from build123d import *

# Parameters (mm, degrees)
MODEL_W            = 2.54
MODEL_H            = 30.48
MODEL_H_2          = 20.32
MODEL_W_2          = 5.08
MODEL_H_3          = 5.08
BOSS_EXTRU_1_DEPTH = 1.5


with BuildPart() as part:
    # Model → Boss.-Extru.1 (new body)
    with BuildSketch(Plane.XY):
        with BuildLine():
            Line((110.49, -34.813931), (110.49, -38.623931))
            Line((110.49, -38.623931), (110.49, -39.893931))
            Line((110.49, -39.893931), (110.49, -123.713931))
            add(Edge.make_bspline(
                [(109.746051, -125.509982), (110.222394, -125.03364), (110.49, -124.387581), (110.49, -123.713931)],
                knots=[0, 0, 0, 0, 1, 1, 1, 1], degree=3))
            add(Edge.make_bspline(
                [(107.95, -126.253931), (108.62365, -126.253931), (109.269709, -125.986325), (109.746051, -125.509982)],
                knots=[0, 0, 0, 0, 1, 1, 1, 1], degree=3))
            Line((107.95, -126.253931), (85.09, -126.253931))
            add(Edge.make_bspline(
                [(83.293949, -125.509982), (83.770291, -125.986325), (84.41635, -126.253931), (85.09, -126.253931)],
                knots=[0, 0, 0, 0, 1, 1, 1, 1], degree=3))
            add(Edge.make_bspline(
                [(82.55, -123.713931), (82.55, -124.387581), (82.817606, -125.03364), (83.293949, -125.509982)],
                knots=[0, 0, 0, 0, 1, 1, 1, 1], degree=3))
            Line((82.55, -123.713931), (82.55, -39.893931))
            Line((82.55, -39.893931), (82.55, -38.623931))
            Line((82.55, -38.623931), (82.55, -34.813931))
            add(Edge.make_bspline(
                [(82.921974, -33.915905), (82.683803, -34.154076), (82.55, -34.477106), (82.55, -34.813931)],
                knots=[0, 0, 0, 0, 1, 1, 1, 1], degree=3))
            add(Edge.make_bspline(
                [(83.82, -33.543931), (83.483175, -33.543931), (83.160146, -33.677734), (82.921974, -33.915905)],
                knots=[0, 0, 0, 0, 1, 1, 1, 1], degree=3))
            Line((83.82, -33.543931), (109.22, -33.543931))
            add(Edge.make_bspline(
                [(110.118026, -33.915905), (109.879854, -33.677734), (109.556825, -33.543931), (109.22, -33.543931)],
                knots=[0, 0, 0, 0, 1, 1, 1, 1], degree=3))
            add(Edge.make_bspline(
                [(110.49, -34.813931), (110.49, -34.477106), (110.356197, -34.154076), (110.118026, -33.915905)],
                knots=[0, 0, 0, 0, 1, 1, 1, 1], degree=3))
        make_face()
        with Locations((107.95, -95.138931)):
            Rectangle(MODEL_W, MODEL_H, mode=Mode.SUBTRACT)
        with Locations((85.09, -90.058931)):
            Rectangle(MODEL_W, MODEL_H_2, mode=Mode.SUBTRACT)
        with Locations((93.98, -105.933931)):
            Rectangle(MODEL_W_2, MODEL_H_3, mode=Mode.SUBTRACT)
        with BuildLine():
            add(Edge.make_bspline(
                [(109.22, -36.083931), (109.22, -36.537658), (108.977939, -36.956919), (108.585, -37.183783)],
                knots=[0, 0, 0, 0, 1, 1, 1, 1], degree=3))
            add(Edge.make_bspline(
                [(108.585, -37.183783), (108.192061, -37.410647), (107.707939, -37.410647), (107.315, -37.183783)],
                knots=[0, 0, 0, 0, 1, 1, 1, 1], degree=3))
            add(Edge.make_bspline(
                [(107.315, -37.183783), (106.922061, -36.956919), (106.68, -36.537658), (106.68, -36.083931)],
                knots=[0, 0, 0, 0, 1, 1, 1, 1], degree=3))
            add(Edge.make_bspline(
                [(106.68, -36.083931), (106.68, -35.630204), (106.922061, -35.210942), (107.315, -34.984079)],
                knots=[0, 0, 0, 0, 1, 1, 1, 1], degree=3))
            add(Edge.make_bspline(
                [(107.315, -34.984079), (107.707939, -34.757215), (108.192061, -34.757215), (108.585, -34.984079)],
                knots=[0, 0, 0, 0, 1, 1, 1, 1], degree=3))
            add(Edge.make_bspline(
                [(108.585, -34.984079), (108.977939, -35.210942), (109.22, -35.630204), (109.22, -36.083931)],
                knots=[0, 0, 0, 0, 1, 1, 1, 1], degree=3))
        make_face(mode=Mode.SUBTRACT)
        with BuildLine():
            add(Edge.make_bspline(
                [(86.36, -36.083931), (86.36, -36.537658), (86.117939, -36.956919), (85.725, -37.183783)],
                knots=[0, 0, 0, 0, 1, 1, 1, 1], degree=3))
            add(Edge.make_bspline(
                [(85.725, -37.183783), (85.332061, -37.410647), (84.847939, -37.410647), (84.455, -37.183783)],
                knots=[0, 0, 0, 0, 1, 1, 1, 1], degree=3))
            add(Edge.make_bspline(
                [(84.455, -37.183783), (84.062061, -36.956919), (83.82, -36.537658), (83.82, -36.083931)],
                knots=[0, 0, 0, 0, 1, 1, 1, 1], degree=3))
            add(Edge.make_bspline(
                [(83.82, -36.083931), (83.82, -35.630204), (84.062061, -35.210942), (84.455, -34.984079)],
                knots=[0, 0, 0, 0, 1, 1, 1, 1], degree=3))
            add(Edge.make_bspline(
                [(84.455, -34.984079), (84.847939, -34.757215), (85.332061, -34.757215), (85.725, -34.984079)],
                knots=[0, 0, 0, 0, 1, 1, 1, 1], degree=3))
            add(Edge.make_bspline(
                [(85.725, -34.984079), (86.117939, -35.210942), (86.36, -35.630204), (86.36, -36.083931)],
                knots=[0, 0, 0, 0, 1, 1, 1, 1], degree=3))
        make_face(mode=Mode.SUBTRACT)
        with BuildLine():
            add(Edge.make_bspline(
                [(86.36, -123.713931), (86.36, -124.167658), (86.117939, -124.586919), (85.725, -124.813783)],
                knots=[0, 0, 0, 0, 1, 1, 1, 1], degree=3))
            add(Edge.make_bspline(
                [(85.725, -124.813783), (85.332061, -125.040647), (84.847939, -125.040647), (84.455, -124.813783)],
                knots=[0, 0, 0, 0, 1, 1, 1, 1], degree=3))
            add(Edge.make_bspline(
                [(84.455, -124.813783), (84.062061, -124.586919), (83.82, -124.167658), (83.82, -123.713931)],
                knots=[0, 0, 0, 0, 1, 1, 1, 1], degree=3))
            add(Edge.make_bspline(
                [(83.82, -123.713931), (83.82, -123.260204), (84.062061, -122.840942), (84.455, -122.614079)],
                knots=[0, 0, 0, 0, 1, 1, 1, 1], degree=3))
            add(Edge.make_bspline(
                [(84.455, -122.614079), (84.847939, -122.387215), (85.332061, -122.387215), (85.725, -122.614079)],
                knots=[0, 0, 0, 0, 1, 1, 1, 1], degree=3))
            add(Edge.make_bspline(
                [(85.725, -122.614079), (86.117939, -122.840942), (86.36, -123.260204), (86.36, -123.713931)],
                knots=[0, 0, 0, 0, 1, 1, 1, 1], degree=3))
        make_face(mode=Mode.SUBTRACT)
        with BuildLine():
            add(Edge.make_bspline(
                [(109.22, -123.713931), (109.22, -124.167658), (108.977939, -124.586919), (108.585, -124.813783)],
                knots=[0, 0, 0, 0, 1, 1, 1, 1], degree=3))
            add(Edge.make_bspline(
                [(108.585, -124.813783), (108.192061, -125.040647), (107.707939, -125.040647), (107.315, -124.813783)],
                knots=[0, 0, 0, 0, 1, 1, 1, 1], degree=3))
            add(Edge.make_bspline(
                [(107.315, -124.813783), (106.922061, -124.586919), (106.68, -124.167658), (106.68, -123.713931)],
                knots=[0, 0, 0, 0, 1, 1, 1, 1], degree=3))
            add(Edge.make_bspline(
                [(106.68, -123.713931), (106.68, -123.260204), (106.922061, -122.840942), (107.315, -122.614079)],
                knots=[0, 0, 0, 0, 1, 1, 1, 1], degree=3))
            add(Edge.make_bspline(
                [(107.315, -122.614079), (107.707939, -122.387215), (108.192061, -122.387215), (108.585, -122.614079)],
                knots=[0, 0, 0, 0, 1, 1, 1, 1], degree=3))
            add(Edge.make_bspline(
                [(108.585, -122.614079), (108.977939, -122.840942), (109.22, -123.260204), (109.22, -123.713931)],
                knots=[0, 0, 0, 0, 1, 1, 1, 1], degree=3))
        make_face(mode=Mode.SUBTRACT)
    extrude(amount=BOSS_EXTRU_1_DEPTH)


solid = part.part
The model under review builds one solid part; all positions refer to its coordinate system, in mm. A direction names the side the tool comes from. Coordinates: 2 decimals unless noted, no trailing zeros. Write each loop counter-clockwise with the first axis right and the second up, starting at its lowest first coordinate (ties: lowest second). Pieces come first, ordered by that corner, then holes. Notation, with made-up numbers: (18.5, 3.25) -> (41.5, 3.25) arc R28 cw to (41.5, 41.25) -> close; hole circle Ø10 at (-27.75, 29.5). An arc over 180 degrees is marked (long way). Answer in a Markdown table with one row per item.
1. Wall thickness on probe 1 along X at (y, z) = (-106, 0.55); probe 2 along Y at (x, z) = (109, 1.4); probe 3 along X at (y, z) = (-100, 1.3): over which ranges is each line inside the solid? List them lowest first. Write a range as [from, to].
Answers below:
| item | result |
|---|---|
| probe 1 | x = [82.55, 91.44], [96.52, 106.68], [109.22, 110.49] |
| probe 2 | y = [-126.03, -124.43], [-123, -110.38], [-79.9, -36.8], [-35.37, -33.54] |
| probe 3 | x = [82.55, 83.82], [86.36, 106.68], [109.22, 110.49] |
2. For faces 1 (the flat face through (96, -33.544, 1)), 2 (the flat face through (108, -110.379, 1)), list the 3-axis set-ups (+Z, -Z, +X, -X, +Y, -Y) from which the entire face can be reached by the end or side of a thin tool; tool diameter is ignored.
Answers below:
| item | result |
|---|---|
| face 1 | +Z, -Z, +X, -X, +Y |
| face 2 | +Z, -Z |
3. Draft analysis for pull direction Y (two halves, no side actions). For faces 3 (the flat face through (82.55, -80, 1)), 4 (the flat face through (97, -126.254, 1)), 5 (the flat face through (85, -100.219, 1)), state which applies: +Y half, -Y half, draft (parallel to the pull), parting line (faces both ways), or undercut.
Answers below:
| item | result |
|---|---|
| face 3 | draft |
| face 4 | -Y half |
| face 5 | undercut |
4. Clearance check with a flat-ended pin moving along its axis: pin 1 Ø12 at (x, y) = (89.5, -65.5) entering from -Z. State where the tip first meets the part, or that it passes through.
Answers below:
| item | result |
|---|---|
| pin 1 | stops at z = 0 |
5. We need section A-A, the plane x = 95. State the section outline as (y, z) points.
Answers below:
| item | result |
|---|---|
| outline | (-126.25, 0) -> (-108.47, 0) -> (-108.47, 1.5) -> (-126.25, 1.5) -> close; (-103.39, 0) -> (-33.54, 0) -> (-33.54, 1.5) -> (-103.39, 1.5) -> close |
6. We need section B-B, the plane z = 0.8. Give the number of separate pieces and of enclosed holes in the cut face, and give its area (3 significant figures).
Answers below:
| item | result |
|---|---|
| separate pieces | 1 |
| enclosed holes | 7 |
| area | 2,410 mm^2 |
